Drawing for the job (mm, zero at the part's lowest x, y, z). Give positions to 0.01 mm unless a question says otherwise; leave off trailing zeros. Write each loop counter-clockwise with the first axis right and the second up, starting at its lowest first coordinate (ties: lowest second). Pieces come first, ordered by that corner, then holes.
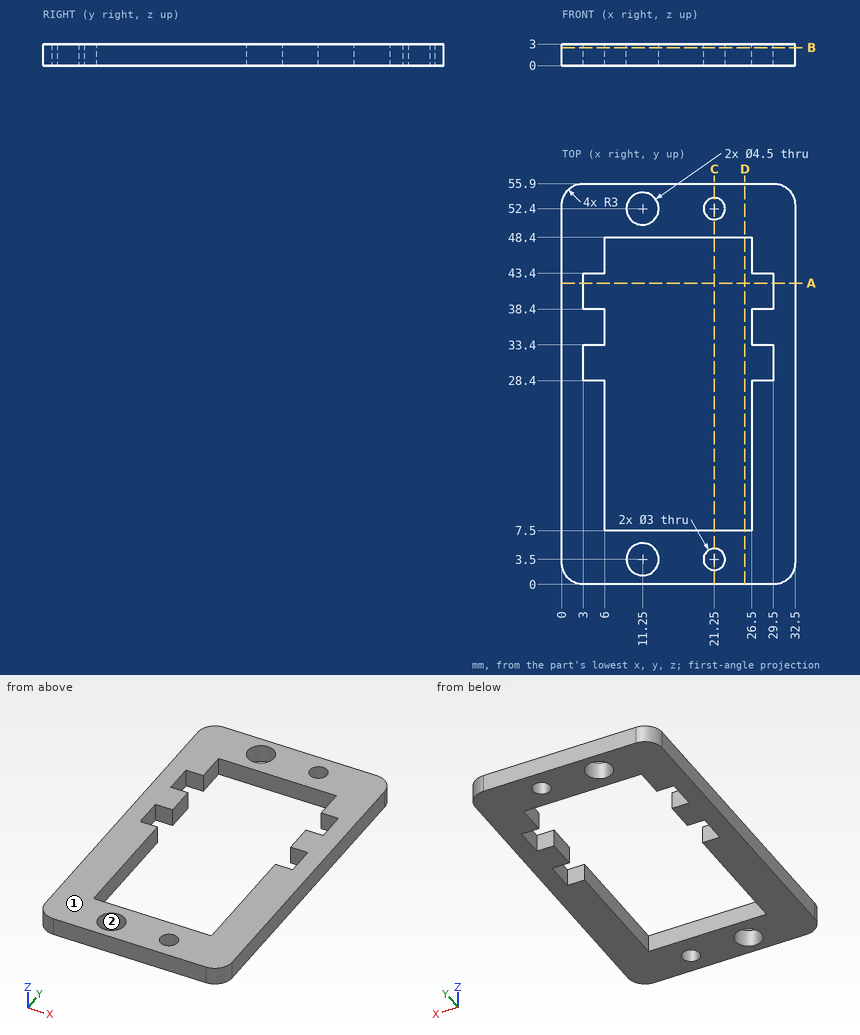
1. Slice it at A-A, the plane y = 42. Write the cut outline in (x, z).
Calculated:
outline: (0, 0) - (3, 0) - (3, 3) - (0, 3) - close; (29.5, 0) - (32.5, 0) - (32.5, 3) - (29.5, 3) - close
2. Pin check, flat tip, straight feed: P1, Ø10, axis at x = 18, y = 26.5, coming from the -Z side. Stop position of the tip, or through.
Calculated:
P1: passes through
3. Slice it at B-B, the plane z = 2.5. State how many separate pieces and enclosed holes the cut face has, and give its area (3 significant figures).
Calculated:
separate pieces: 1
enclosed holes: 5
area: 865 mm2
4. Slice it at C-C, the plane x = 21.25. Write the cut outline in (y, z).
Calculated:
outline: (0, 0) - (2, 0) - (2, 3) - (0, 3) - close; (5, 0) - (7.5, 0) - (7.5, 3) - (5, 3) - close; (48.4, 0) - (50.9, 0) - (50.9, 3) - (48.4, 3) - close; (53.9, 0) - (55.9, 0) - (55.9, 3) - (53.9, 3) - close
5. Slice it at D-D, the plane x = 25.5. Write the cut outline in (y, z), and give its area (3 significant figures).
Calculated:
outline: (0, 0) - (7.5, 0) - (7.5, 3) - (0, 3) - close; (48.4, 0) - (55.9, 0) - (55.9, 3) - (48.4, 3) - close
area: 45.0 mm2
6. Pull direction X, two halves, no side cores. Call the marked faces 1 and 2: +X half, -X half, draft (parallel to the pull), parting line (faces both ways), or undercut.
Calculated:
face 1: draft
face 2: undercut
7. Probe probe 1 along Y at (x, z) = (11.25, 1.35); probe 2 along X at (y, z) = (3.5, 0.8); probe 3 along Y at (x, z) = (21.25, 0.95). List the from-to ranges inside material, lowest first.
Calculated:
probe 1: y = 0 to 1.25, 5.75 to 7.5, 48.4 to 50.15, 54.65 to 55.9
probe 2: x = 0 to 9, 13.5 to 19.75, 22.75 to 32.5
probe 3: y = 0 to 2, 5 to 7.5, 48.4 to 50.9, 53.9 to 55.9
